```python
from build123d import *

# Parameters (mm, degrees)
F3_DEPTH = 1.5875
F1_R     = 1.5875
F1_R_2   = 3.175
F4_DEPTH = 12.7


with BuildPart() as f3:
    # F0 (on Right) → F3 (new body, symmetric)
    with BuildSketch(Plane.YZ):
        Polygon((57.15, 4.75869), (57.15, 46.04131), (-107.95, 46.04131), (-107.95, 20.64131), (-28.575, 4.75869), align=None)
    extrude(amount=F3_DEPTH, both=True)

    # F1 (on Right) → F4 (cut, symmetric)
    with BuildSketch(Plane.YZ):
        with Locations((19.05, 20.63369)):
            Circle(F1_R)
        with Locations((-63.5, 36.50869)):
            Circle(F1_R_2)
    extrude(amount=F4_DEPTH, both=True, mode=Mode.SUBTRACT)


solid = f3.part
```
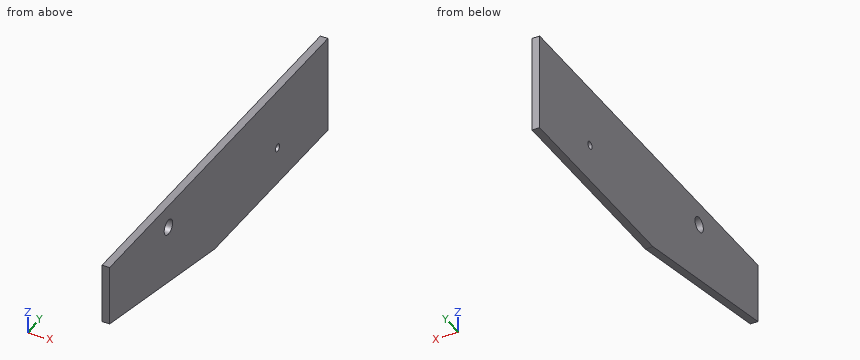
The listing builds one solid part. Answer for the finished solid, in the listing's coordinates (mm). Give positions to 0.01 mm unless a question says otherwise; leave off trailing zeros. Order: outer loops, then holes, each group sorted by start corner. A loop starts at its lowest first (then second) coordinate and runs counter-clockwise, first axis right, second up. Notation, with made-up numbers: (46.5, -34) - (64.5, -34) arc R37 ccw to (64.5, 3) - close; hole circle Ø7 at (-13.5, 59). An arc over 180 degrees is marked (long way). Answer in a Markdown table with one row per item. Add a question column.
Q1. Given P1, Ø3, axis at y = 19.05, z = 20.63, coming from the +X side, flat-ended and moving along its own axis, determine where the tip first touches the part or whether it passes through.
Q2. The part is cut by section D-D (y = -34). Determine the outline of the cut face in (x, z), then the cut area to 3 significant figures.
Q3. Find the intervals of material crossed by line 1 along Z through (x, y) = (0.4, 19.05); line 2 along Y through (x, z) = (-0.4, 37.5); line 3 along Z through (x, y) = (0.5, -63.5), in increasing order. Write a range as [from, to].
Q4. The part is cut by section A-A (y = -63.5). Determine the outline of the cut face in (x, z).
Q5. The part is cut by section B-B (x = -0.7). Give the number of separate pieces and of enclosed holes in the cut face, then the cut area to 3 significant figures.
Q6. The part is cut by section C-C (y = 19.05). Determine the outline of the cut face in (x, z).
Determined:
| question | item | result |
|---|---|---|
| 1 | P1 | passes through |
| 2 | outline | (-1.59, 5.84) - (1.59, 5.84) - (1.59, 46.04) - (-1.59, 46.04) - close |
| 2 | area | 128 mm² |
| 3 | line 1 | z = [4.76, 19.05], [22.22, 46.04] |
| 3 | line 2 | y = [-107.95, -66.52], [-60.48, 57.15] |
| 3 | line 3 | z = [11.75, 33.33], [39.68, 46.04] |
| 4 | outline | (-1.59, 11.75) - (1.59, 11.75) - (1.59, 33.33) - (-1.59, 33.33) - close; (-1.59, 39.68) - (1.59, 39.68) - (1.59, 46.04) - (-1.59, 46.04) - close |
| 5 | separate pieces | 1 |
| 5 | enclosed holes | 2 |
| 5 | area | 6,150 mm² |
| 6 | outline | (-1.59, 4.76) - (1.59, 4.76) - (1.59, 19.05) - (-1.59, 19.05) - close; (-1.59, 22.22) - (1.59, 22.22) - (1.59, 46.04) - (-1.59, 46.04) - close |
